from build123d import *

# Parameters (mm, degrees)
F1_DEPTH = 8
F2_T     = -1
F4_DEPTH = 1
F6_R     = 1.5
F7_DEPTH = 8.001


with BuildPart() as f1:
    # F0 (on Top) → F1 (new body)
    with BuildSketch(Plane.XY):
        with BuildLine():
            Line((-13.65, -7.45), (13.65, -7.45))
            ThreePointArc((13.65, -7.45), (15.77132, -6.57132), (16.65, -4.45))
            Line((16.65, -4.45), (16.65, 4.45))
            ThreePointArc((16.65, 4.45), (15.77132, 6.57132), (13.65, 7.45))
            Line((13.65, 7.45), (-13.65, 7.45))
            ThreePointArc((-13.65, 7.45), (-15.77132, 6.57132), (-16.65, 4.45))
            Line((-16.65, 4.45), (-16.65, -4.45))
            ThreePointArc((-16.65, -4.45), (-15.77132, -6.57132), (-13.65, -7.45))
        make_face()
    extrude(amount=F1_DEPTH)

    # F2
    f2_openings = [f1.faces().sort_by_distance(p)[0] for p in [
        (0, 0, 8),
    ]]
    offset(amount=F2_T, openings=f2_openings)


with BuildPart() as f4:
    # F3 (on face) → F4 (new body)
    with BuildSketch(Plane(origin=(0, 0, 0), x_dir=(1, 0, 0), z_dir=(0, 0, -1))):
        with BuildLine():
            Line((-14.5, -8.25), (14.5, -8.25))
            ThreePointArc((14.5, -8.25), (16.62132, -7.37132), (17.5, -5.25))
            Line((17.5, -5.25), (17.5, 5.25))
            ThreePointArc((17.5, 5.25), (16.62132, 7.37132), (14.5, 8.25))
            Line((14.5, 8.25), (-14.5, 8.25))
            ThreePointArc((-14.5, 8.25), (-16.62132, 7.37132), (-17.5, 5.25))
            Line((-17.5, 5.25), (-17.5, -5.25))
            ThreePointArc((-17.5, -5.25), (-16.62132, -7.37132), (-14.5, -8.25))
        make_face()
        with BuildLine():
            Line((-13.65, 7.45), (13.65, 7.45))
            ThreePointArc((13.65, 7.45), (15.77132, 6.57132), (16.65, 4.45))
            Line((16.65, 4.45), (16.65, -4.45))
            ThreePointArc((16.65, -4.45), (15.77132, -6.57132), (13.65, -7.45))
            Line((13.65, -7.45), (-13.65, -7.45))
            ThreePointArc((-13.65, -7.45), (-15.77132, -6.57132), (-16.65, -4.45))
            Line((-16.65, -4.45), (-16.65, 4.45))
            ThreePointArc((-16.65, 4.45), (-15.77132, 6.57132), (-13.65, 7.45))
        make_face(mode=Mode.SUBTRACT)
    extrude(amount=-F4_DEPTH)


with BuildPart() as f1_1:
    add(f1.part)

    # F5: union F4
    add(f4.part)

    # F6 (on face) → F7 (cut, through all)
    with BuildSketch(Plane(origin=(0, 0, 0), x_dir=(1, 0, 0), z_dir=(0, 0, -1))):
        with Locations((-2.5, 0.25)):
            Circle(F6_R)
        with Locations((2.5, 0.25)):
            Circle(F6_R)
    extrude(amount=-F7_DEPTH, mode=Mode.SUBTRACT)


solid = f1_1.part
Build history of the part. All positions in model axes, mm. A direction names the side the tool comes from. Coordinates: 2 decimals unless noted, no trailing zeros. Write each loop counter-clockwise with the first axis right and the second up, starting at its lowest first coordinate (ties: lowest second). Pieces come first, ordered by that corner, then holes.
(1) Mould opens along Y. For faces 5 (the cylindrical face through (15.75, -6.59, 4.45)), 6 (the flat face through (0, -8, 1)), 7 (the flat face through (-15.65, 0, 4)), 8 (the cylindrical face through (15.08, 5.85, 4.45)) say: pulls with the +Y half, pulls with the -Y half, needs draft (parallel to the pull), parting line crosses it, or undercut.
(2) Cut at D-D on y = 3.25. List the corners of the cut face in (x, z), and give its area (3 significant figures).
(3) 3-axis set-ups, long thin cutter, end or side, ignore diameter. For faces 1 (the flat face through (0, 7.45, 4)), 2 (the cylindrical face through (-15.75, 6.59, 4.45)), 3 (the flat face through (0, -7.45, 4)), 4 (the flat face through (0, 6.45, 4)): which of +Z, -Z, +X, -X, +Y, -Y reach the whole face in a straight line?
(4) Cut at A-A on x = -2.5. List the corners of the cut face in (y, z).
(5) Cut at C-C on z = 6. List the corners of the cut face in (x, y).
(6) Pin check, flat tips, straight feed: pin 1 Ø2 at (x, y) = (-9.5, -2) entering from +Z; pin 2 Ø3 at (y, z) = (5, 4) entering from +X; pin 3 Ø2 at (x, z) = (5.5, 3.5) entering from +Y; pin 4 Ø1.8 at (x, y) = (2.5, -0.25) entering from +Z. Stop position of each tip, or through.
(7) Cut at B-B on y = -0.25. List the corners of the cut face in (x, z), and give its area (3 significant figures).
(8) Drill centre lines: line 1 (X direction, y = -0.25, z = 0.55); line 2 (Y direction, x = 13.5, z = 2.5); line 3 (Y direction, x = -2.5, z = 0.5). Where is each one in solid material? Low to high.
Working result:
1. face 5: pulls with the -Y half
1. face 6: needs draft
1. face 7: undercut
1. face 8: undercut
2. outline: (-17.5, 0) - (17.5, 0) - (17.5, 1) - (16.65, 1) - (16.65, 8) - (15.65, 8) - (15.65, 1) - (-15.65, 1) - (-15.65, 8) - (-16.65, 8) - (-16.65, 1) - (-17.5, 1) - close
2. area: 49.0 mm2
3. face 1: +Z, +X, -X, +Y
3. face 2: +Z, -X, +Y
3. face 3: +Z, +X, -X, -Y
3. face 4: +Z
4. outline: (-8.25, 0) - (-1.75, 0) - (-1.75, 1) - (-6.45, 1) - (-6.45, 8) - (-7.45, 8) - (-7.45, 1) - (-8.25, 1) - close; (1.25, 0) - (8.25, 0) - (8.25, 1) - (7.45, 1) - (7.45, 8) - (6.45, 8) - (6.45, 1) - (1.25, 1) - close
5. outline: (-16.65, -4.45) arc R3 ccw to (-13.65, -7.45) - (13.65, -7.45) arc R3 ccw to (16.65, -4.45) - (16.65, 4.45) arc R3 ccw to (13.65, 7.45) - (-13.65, 7.45) arc R3 ccw to (-16.65, 4.45) - close; hole (-15.65, -4.45) arc R2 ccw to (-13.65, -6.45) - (13.65, -6.45) arc R2 ccw to (15.65, -4.45) - (15.65, 4.45) arc R2 ccw to (13.65, 6.45) - (-13.65, 6.45) arc R2 ccw to (-15.65, 4.45) - close
6. pin 1: stops at z = 1
6. pin 2: stops at x = 16.65
6. pin 3: stops at y = 7.45
6. pin 4: passes through
7. outline: (-17.5, 0) - (-4, 0) - (-4, 1) - (-15.65, 1) - (-15.65, 8) - (-16.65, 8) - (-16.65, 1) - (-17.5, 1) - close; (-1, 0) - (1, 0) - (1, 1) - (-1, 1) - close; (4, 0) - (17.5, 0) - (17.5, 1) - (16.65, 1) - (16.65, 8) - (15.65, 8) - (15.65, 1) - (4, 1) - close
7. area: 43.0 mm2
8. line 1: x = -17.5 to -4, -1 to 1, 4 to 17.5
8. line 2: y = -7.45 to -6.45, 6.45 to 7.45
8. line 3: y = -8.25 to -1.75, 1.25 to 8.25
